Build history of the part. All positions in model axes, mm. A direction names the side the tool comes from. Round coordinates to 2 decimals unless told otherwise and drop trailing zeros. Write each loop counter-clockwise with the first axis right and the second up, starting at its lowest first coordinate (ties: lowest second). Pieces come first, ordered by that corner, then holes. Notation, with made-up numbers: (-15.75, 11.5) - (19.25, 11.5) arc R26 cw to (19.25, 28.5) - close; hole circle Ø3 at (57, -2.75). An arc over 180 degrees is marked (long way). Answer as a JSON object with one key per item and string values. Group by question number.
Item 1: Slice it at C-C, the plane x = 0. List the corners of the cut face in (y, z), then the cut area to 3 significant figures.
Item 2: Which spindle directions (+Z, -Z, +X, -X, +Y, -Y) get a long thin tool onto all of the face, cutting with end or side? Do faces 4 (the flat face through (-33.1, 2.6, -7.5)), 5 (the cylindrical face through (-0.29, 43.23, -4.93)). Say none if no direction does.
Item 3: Slice it at B-B, the plane y = 0. List the corners of the cut face in (x, z).
Item 4: Slice it at A-A, the plane x = -15. List the corners of the cut face in (y, z), then the cut area to 3 significant figures.
Item 5: Flat gauge pins, fed straight in: pin 1 (6 mm diameter, centred on y = -13, z = -7.5, fed in from -X); pin 2 (2 mm diameter, centred on x = -28, z = -6.5, fed in from +Y); pin 3 (1.5 mm diameter, centred on y = 34.5, z = -2, fed in from +X). Where does each tip first touch, or does it go through?
Item 6: Probe line 1 (Y direction, x = 0, z = -2.25); line 2 (Y direction, x = 0, z = -8.35); line 3 (X direction, y = 0, z = -2.5). List the from-to ranges inside material, lowest first. Write a range as from..to.
Item 7: Slice it at D-D, the plane y = -20.5. List the corners of the cut face in (x, z).
Item 8: Two-plate mould, pull along Y, no slides. Class faces 1 (the cylindrical face through (20.765, 39.923, -4.93)), 2 (the cylindrical face through (30.5, 12.6, -8.8)), 3 (the flat face through (-37, -4, 0)): +Y half, -Y half, draft (parallel to the pull), parting line (faces both ways), or undercut.
from build123d import *

# Parameters (mm, degrees)
ESQUISSE2_R                  = 2.25
ENL_V_MAT_EXTRU_1_DEPTH      = 65.420493634
R_P_TITION_CIRCULAIRE1_COUNT = 3


with BuildPart() as part:
    # Esquisse1 → Base-Révolution (revolve)
    with BuildSketch(Plane(origin=(0, 0, 0), x_dir=(1, 0, 0), z_dir=(0, 1, 0))):
        Polygon((33, 10), (45, 10), (45, 0), (37, 0), (37, 7.5), (33, 7.5), align=None)
    revolve(axis=Axis((0, 0, 30), (0, 0, -1)))

    # Esquisse2 → Enlèv. mat.-Extru.1 (cut, through all)
    with BuildSketch(Plane.XY):
        with Locations((0, 41)):
            Circle(ESQUISSE2_R)
    enl_v_mat_extru_1 = extrude(amount=-ENL_V_MAT_EXTRU_1_DEPTH, mode=Mode.SUBTRACT)

    # Répétition circulaire1: Enlèv. mat.-Extru.1 ×3 about axis
    r_p_tition_circulaire1_axis = Axis((0, 0, 0), (0, 0, 1))
    for i in range(1, R_P_TITION_CIRCULAIRE1_COUNT):
        add(enl_v_mat_extru_1.rotate(r_p_tition_circulaire1_axis, i * 360 / R_P_TITION_CIRCULAIRE1_COUNT), mode=Mode.SUBTRACT)


solid = part.part
Geometry says:
{
 "1": {"outline": "(-45, -10) - (-33, -10) - (-33, -7.5) - (-37, -7.5) - (-37, 0) - (-45, 0) - close; (33, -10) - (38.75, -10) - (38.75, 0) - (37, 0) - (37, -7.5) - (33, -7.5) - close; (43.25, -10) - (45, -10) - (45, 0) - (43.25, 0) - close", "area": "135 mm^2"},
 "2": {"face 4": "+Z", "face 5": "+Z, -Z"},
 "3": {"outline": "(-45, -10) - (-33, -10) - (-33, -7.5) - (-37, -7.5) - (-37, 0) - (-45, 0) - close; (33, -10) - (45, -10) - (45, 0) - (37, 0) - (37, -7.5) - (33, -7.5) - close"},
 "4": {"outline": "(-42.43, -10) - (-29.39, -10) - (-29.39, -7.5) - (-33.82, -7.5) - (-33.82, 0) - (-42.43, 0) - close; (29.39, -10) - (42.43, -10) - (42.43, 0) - (33.82, 0) - (33.82, -7.5) - (29.39, -7.5) - close", "area": "194 mm^2"},
 "5": {"pin 1": "stops at x = -43.87", "pin 2": "stops at y = 36", "pin 3": "stops at x = 29.76"},
 "6": {"line 1": "y = -45..-37, 37..38.75, 43.25..45", "line 2": "y = -45..-33, 33..38.75, 43.25..45", "line 3": "x = -45..-37, 37..45"},
 "7": {"outline": "(-40.06, -10) - (-37.76, -10) - (-37.76, 0) - (-40.06, 0) - close; (-33.26, -10) - (-25.86, -10) - (-25.86, -7.5) - (-30.8, -7.5) - (-30.8, 0) - (-33.26, 0) - close; (25.86, -10) - (33.26, -10) - (33.26, 0) - (30.8, 0) - (30.8, -7.5) - (25.86, -7.5) - close; (37.76, -10) - (40.06, -10) - (40.06, 0) - (37.76, 0) - close"},
 "8": {"face 1": "parting line", "face 2": "undercut", "face 3": "draft"}
}
